```python
from build123d import *

# Parameters (mm, degrees)
F0_W     = 51
F0_H     = 48
F0_R     = 4.5
F0_R_2   = 2
F0_W_2   = 11.5
F0_H_2   = 20
F1_DEPTH = 2
F3_DEPTH = 6
F4_W     = 1
F4_H     = 12
F5_DEPTH = 3
F6_R     = 5
F7_R     = 0.99999
F8_R     = 10


# Not quite as in the source:
# - a fillet or chamfer is up to 0.001 mm smaller than in the source, because OpenCascade refuses the exact size


with BuildPart() as f1:
    # F0 (on Top) → F1 (new body)
    with BuildSketch(Plane.XY):
        with Locations((25.5, 24)):
            Rectangle(F0_W, F0_H)
        with Locations((10.25, 13.5)):
            Circle(F0_R, mode=Mode.SUBTRACT)
        with Locations((10.25, 22.5)):
            Circle(F0_R_2, mode=Mode.SUBTRACT)
        with Locations((45.25, 6)):
            Circle(F0_R_2, mode=Mode.SUBTRACT)
        with Locations((28.75, 22.5)):
            Rectangle(F0_W_2, F0_H_2, mode=Mode.SUBTRACT)
        with Locations((10.25, 31.5)):
            Circle(F0_R, mode=Mode.SUBTRACT)
        with Locations((45.25, 39)):
            Circle(F0_R_2, mode=Mode.SUBTRACT)
    extrude(amount=F1_DEPTH)

    # F2 (on face) → F3 (join)
    with BuildSketch(Plane(origin=(0, 48, 0), x_dir=(-1, 0, 0), z_dir=(0, 1, 0))):
        Polygon((-10, 2), (-41, 2), (-41, 0), (-41, -10), (-10, -10), (-10, 0), align=None)
    extrude(amount=F3_DEPTH)

    # F4 (on face) → F5 (cut)
    with BuildSketch(Plane(origin=(0, 54, 0), x_dir=(-1, 0, 0), z_dir=(0, 1, 0))):
        with Locations((-20, -4)):
            Rectangle(F4_W, F4_H)
        with Locations((-31, -4)):
            Rectangle(F4_W, F4_H)
    extrude(amount=-F5_DEPTH, mode=Mode.SUBTRACT)

    # F6
    f6_edges = [f1.edges().sort_by_distance(p)[0] for p in [
        (10, 48, 1),
        (41, 48, 1),
    ]]
    fillet(f6_edges, radius=F6_R)

    # F7 (radius 1 in the source; OpenCascade refuses exactly that, so slightly less here)
    f7_edges = [f1.edges().sort_by_distance(p)[0] for p in [
        (41, 54, -4),
        (10, 54, -4),
        (10, 51, -10),
        (41, 51, -10),
    ]]
    fillet(f7_edges, radius=F7_R)

    # F8
    f8_edges = [f1.edges().sort_by_distance(p)[0] for p in [
        (51, 48, 1),
        (0, 48, 1),
        (51, 0, 1),
    ]]
    fillet(f8_edges, radius=F8_R)


solid = f1.part
```
Verification items for the finished model (mm, model axes). A direction names the side the tool comes from. Round coordinates to 2 decimals unless told otherwise and drop trailing zeros. Order: outer loops, then holes, each group sorted by start corner. A loop starts at its lowest first (then second) coordinate and runs counter-clockwise, first axis right, second up. Notation, with made-up numbers: (30.25, 77.5) - (40.25, 77.5) arc R27 ccw to (40.25, 101.5) - close; hole circle Ø3 at (30, 48). An arc over 180 degrees is marked (long way). Use CSV: the item, a comma, the result in double quotes. Start each with the question number.
1) Section check C-C, the plane y = 6. Record the cut outline in (x, z).
2) Section check D-D, the plane x = 46.5. State how many separate pieces and enclosed holes the cut face has, plus the area to 3 significant figures.
3) Thickness scan on L1, parallel to Y at x = 10.25, z = 1.4; L2, parallel to Y at x = 9, z = 1.25; L3, parallel to Y at x = 45.25, z = 0.9. Record the ranges inside material, lowest first.
4) Mould release check, pull along X, two halves, no side actions. Record for faces 6 (the flat face through (41, 50, -5)), 7 (the flat face through (36, 54, -4)), 8 (the cylindrical face through (44.816, 37.048, 0.986)): +X half, -X half, draft (parallel to the pull), parting line (faces both ways), or undercut.
5) Section check B-B, the plane z = -4.5. Record the cut outline in (x, y).
6) Go/stop test with flat-tipped pins: P1, Ø4.5, axis at x = 45.25, y = 6, coming from the +Z side; P2, Ø15.5, axis at x = 16.5, y = 14, coming from the -Z side; P3, Ø0.8, axis at x = 20, z = -2, coming from the +Y side; P4, Ø2.5, axis at y = 50, z = -5, coming from the +X side. Record where each tip stops, or that it passes through.
7) Access from +Z, -Z, +X, -X, +Y, -Y to the whole of each face (thin tool, end or side, straight path). Record for faces 1 (the flat face through (20.5, 53, -4)), 2 (the flat face through (29, 32.5, 1)), 3 (the cylindrical face through (47.99, 2.85, 1.01)), 4 (the flat face through (19, 27, 2)), 5 (the flat face through (10, 50, -5)).
8) Section check A-A, the plane y = 13.5. Record the cut outline in (x, z).
Answers:
1,outline,"(0, 0) - (43.25, 0) - (43.25, 2) - (0, 2) - close; (47.25, 0) - (50.17, 0) - (50.17, 2) - (47.25, 2) - close"
2,separate pieces,"3"
2,enclosed holes,"0"
2,area,"78.6 mm²"
3,L1,"y = 0 to 9, 18 to 20.5, 24.5 to 27, 36 to 53.66"
3,L2,"y = 0 to 9.18, 17.82 to 20.94, 24.06 to 27.18, 35.82 to 50"
3,L3,"y = 0.95 to 4, 8 to 37, 41 to 47.91"
4,face 6,"+X half"
4,face 7,"draft"
4,face 8,"undercut"
5,outline,"(10, 48) - (41, 48) - (41, 53) arc R1 ccw to (40, 54) - (31.5, 54) - (31.5, 51) - (30.5, 51) - (30.5, 54) - (20.5, 54) - (20.5, 51) - (19.5, 51) - (19.5, 54) - (11, 54) arc R1 ccw to (10, 53) - close"
6,P1,"stops at z = 2"
6,P2,"stops at z = 0"
6,P3,"stops at y = 51"
6,P4,"stops at x = 41"
7,face 1,"+Z, -Z, +Y"
7,face 2,"+Z, -Z"
7,face 3,"+Z, -Z, +X, -Y"
7,face 4,"+Z, +X, -X, +Y, -Y"
7,face 5,"-Z, -X, +Y, -Y"
8,outline,"(0, 0) - (5.75, 0) - (5.75, 2) - (0, 2) - close; (14.75, 0) - (23, 0) - (23, 2) - (14.75, 2) - close; (34.5, 0) - (51, 0) - (51, 2) - (34.5, 2) - close"
